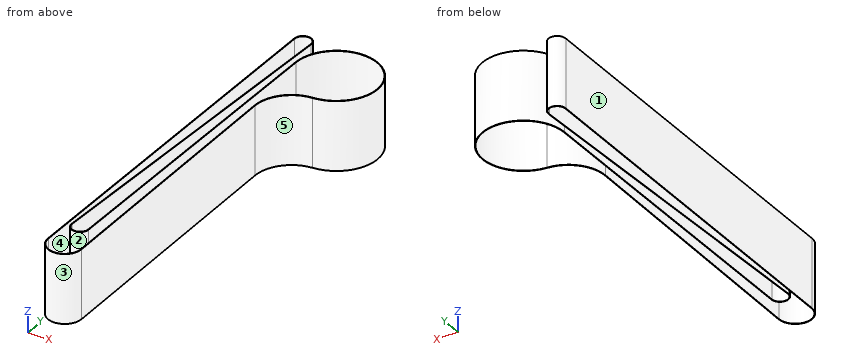
```python
from build123d import *

# Parameters (mm, degrees)
BOSS_EXTRUDE1_DEPTH = 34


with BuildPart() as part:
    # Sketch1 → Boss-Extrude1 (new body)
    with BuildSketch(Plane.XY):
        with BuildLine():
            Line((3.746, 15), (3.746, 43))
            Line((3.746, 43), (3.746, 173))
            Line((3.746, 173), (3.746, 205))
            ThreePointArc((3.746, 205), (8.076040586, 209.25332033), (12.251281537, 204.847943126))
            Line((12.251281537, 204.847943126), (6.002556148, 30.142977785))
            ThreePointArc((6.002556148, 30.142977785), (9.922734835, 26.000746308), (13.999983378, 29.988468323))
            Line((13.999983378, 29.988468323), (14.459106014, 189.24396707))
            ThreePointArc((14.459106014, 189.24396707), (48.621297679, 203.909175827), (35.923887521, 168.967804038))
            ThreePointArc((35.923887521, 168.967804038), (23.840329441, 163.281004469), (19.000766489, 150.833888513))
            Line((19.000766489, 150.833888513), (20.253648522, 15.076171345))
            ThreePointArc((20.253648522, 15.076171345), (12.038086078, 6.74608787), (3.746, 15))
        make_face()
        with BuildLine():
            Line((4, 43), (4, 173))
            Line((4, 173), (4, 205))
            ThreePointArc((4, 205), (8.071500316, 208.999360912), (11.997443852, 204.857022215))
            Line((11.997443852, 204.857022215), (5.748718463, 30.152056874))
            ThreePointArc((5.748718463, 30.152056874), (9.917828497, 25.746793698), (14.253982322, 29.987736062))
            Line((14.253982322, 29.987736062), (14.713104958, 189.243234808))
            ThreePointArc((14.713104958, 189.243234808), (48.446877709, 203.724531103), (35.908702378, 169.221349717))
            ThreePointArc((35.908702378, 169.221349717), (23.654631868, 163.454303088), (18.746777305, 150.831544495))
            Line((18.746777305, 150.831544495), (19.999659338, 15.073827328))
            ThreePointArc((19.999659338, 15.073827328), (12.036914057, 7.000085166), (4, 15))
            Line((4, 15), (4, 43))
        make_face(mode=Mode.SUBTRACT)
    extrude(amount=BOSS_EXTRUDE1_DEPTH)


solid = part.part
```
The model under review builds one solid part; all positions refer to its coordinate system, in mm. Face numbers are marked on the shaded views. A direction names the side the tool comes from. Give positions to 0.01 mm unless a question says otherwise; leave off trailing zeros. Write each loop counter-clockwise with the first axis right and the second up, starting at its lowest first coordinate (ties: lowest second). Pieces come first, ordered by that corner, then holes. Notation, with made-up numbers: M 56.25,-1 L 112.25,-1 A30 ccw 112.25,31 Z; hole C 51,18.25 d9. An arc over 180 degrees is marked long. Answer in a Markdown table with one row per item.
Item 1: Draft analysis for pull direction X (two halves, no side actions). For the marked faces 3, 4 and 5, state which applies: +X half, -X half, draft (parallel to the pull), parting line (faces both ways), or undercut.
Check sheet entries:
| item | result |
|---|---|
| face 3 | parting line |
| face 4 | undercut |
| face 5 | +X half |
Item 2: Add section C-C on z = 9.5. Give the boundary of the cut face in (x, y), plus the area to 3 significant figures.
Check sheet entries:
| item | result |
|---|---|
| outline | M 3.75,15 A8.25 ccw long 20.25,15.08 L 19,150.83 A18 cw 35.92,168.97 A20.25 ccw long 14.46,189.24 L 14,29.99 A4 cw long 6,30.14 L 12.25,204.85 A4.25 ccw long 3.75,205 Z; hole M 4,15 A8 ccw long 20,15.07 L 18.75,150.83 A18.25 cw 35.91,169.22 A20 ccw long 14.71,189.24 L 14.25,29.99 A4.25 cw long 5.75,30.15 L 12,204.86 A4 ccw long 4,205 Z |
| area | 212 mm2 |
Item 3: For line 1 along X through (y, z) = (151, 30); line 2 along X through (y, z) = (182, 24); line 3 along Y through (x, z) = (28.5, 31), list the stretches that pass through material, from the lowest coordinate up.
Check sheet entries:
| item | result |
|---|---|
| line 1 | 3.75 to 4, 10.07 to 10.33, 14.35 to 14.6, 18.75 to 19 |
| line 2 | 3.75 to 4, 11.18 to 11.43, 14.44 to 14.69, 53.38 to 53.65 |
| line 3 | 166.87 to 167.15, 208.2 to 208.46 |
Item 4: Tool access review of the marked faces 1 and 2: name each direction out of +Z, -Z, +X, -X, +Y, -Y from which nothing blocks a thin tool from reaching the whole face with its end or side.
Check sheet entries:
| item | result |
|---|---|
| face 1 | +Z, -Z, -X, +Y, -Y |
| face 2 | +Z, -Z |
Item 5: Add section B-B on y = 54. Give the boundary of the cut face in (x, z).
Check sheet entries:
| item | result |
|---|---|
| outline | M 3.75,0 L 4,0 L 4,34 L 3.75,34 Z; M 6.6,0 L 6.86,0 L 6.86,34 L 6.6,34 Z; M 14.07,0 L 14.32,0 L 14.32,34 L 14.07,34 Z; M 19.64,0 L 19.89,0 L 19.89,34 L 19.64,34 Z |
Item 6: Add section A-A on x = 44.5. Give the boundary of the cut face in (y, z), plus the area to 3 significant figures.
Check sheet entries:
| item | result |
|---|---|
| outline | M 171.45,0 L 171.74,0 L 171.74,34 L 171.45,34 Z; M 206.63,0 L 206.92,0 L 206.92,34 L 206.63,34 Z |
| area | 19.8 mm2 |
Item 7: Add section D-D on x = 10. Give the boundary of the cut face in (y, z), plus the area to 3 significant figures.
Check sheet entries:
| item | result |
|---|---|
| outline | M 6.99,0 L 7.25,0 L 7.25,34 L 6.99,34 Z; M 25.75,0 L 26,0 L 26,34 L 25.75,34 Z; M 141.91,0 L 149.01,0 L 149.01,34 L 141.91,34 Z; M 208.46,0 L 208.75,0 L 208.75,34 L 208.46,34 Z |
| area | 269 mm2 |
Item 8: For P1, Ø2, axis at x = 30, z = 13.5, coming from the +Y side; P2, Ø10, axis at x = 22.5, y = 77.5, coming from the +Z side; P3, Ø10, axis at y = 178, z = 28.5, coming from the +X side; P4, Ø5, axis at y = 175.5, z = 23, coming from the +X side, all flat-tipped, find the tip position at first contact; note any pin that passes through.
Check sheet entries:
| item | result |
|---|---|
| P1 | y = 209.1 |
| P2 | z = 34 |
| P3 | x = 54 |
| P4 | x = 51.6 |
